```python
from build123d import *

# Parameters (mm, degrees)
EXTRUDE_1_DEPTH     = 3
SKETCH_2_W          = 112
SKETCH_2_H          = 45
CUT_EXTRUDE_1_DEPTH = 174.386325559


with BuildPart() as part:
    # Эскиз1 → Бобышка-Вытянуть1 (new body)
    with BuildSketch(Plane(origin=(0, 0, 0), x_dir=(1, 0, 0), z_dir=(0, 1, 0))):
        with BuildLine():
            Line((0, 0), (138, 0))
            Line((138, 0), (138, -68))
            ThreePointArc((138, -68), (69, -104.927679336), (0, -68))
            Line((0, -68), (0, 0))
        make_face()
    extrude(amount=EXTRUDE_1_DEPTH)

    # Эскиз2 → Вырез-Вытянуть1 (cut, through all)
    with BuildSketch(Plane(origin=(0, 3, 0), x_dir=(1, 0, 0), z_dir=(0, 1, 0))):
        with Locations((69, -31.5)):
            Rectangle(SKETCH_2_W, SKETCH_2_H)
    extrude(amount=-CUT_EXTRUDE_1_DEPTH, mode=Mode.SUBTRACT)

    # Эскиз3 → Зенковка для  винта с плоской головкой M51 (revolve, cut)
    with BuildSketch(Plane(origin=(69, 3, 82.6), x_dir=(0, 0, 1), z_dir=(1, 0, 0))):
        Polygon((0, 0), (0, 3), (2.75, 3), (2.75, 2.45), (5.2, 0), align=None)
    revolve(axis=Axis((69, 9.35, 82.6), (0, -1, 0)), mode=Mode.SUBTRACT)


solid = part.part
```
CAD build for the part. Positions are in the model's coordinates, mm. A direction names the side the tool comes from. Give positions to 0.01 mm unless a question says otherwise; leave off trailing zeros. Loops run counter-clockwise (first coordinate to the right, second up) from the corner with the lowest first, then second, coordinate; pieces in that order, holes last. Notation, with made-up numbers: M 18,22 L 73,22 A20 ccw 73,33 Z; hole C -8,-35 d6. An arc over 180 degrees is marked long. Use one line per item in the form item = value.
Item 1: Drill centre lines: probe 1 along X at (y, z) = (1, 39.5); probe 2 along Z at (x, y) = (80, 0.6); probe 3 along X at (y, z) = (0.4, 82.6). Where is each one in solid material? Low to high. Write a range as from..to.
Determined:
probe_1 = 0..13, 125..138
probe_2 = 0..9, 54..104.19
probe_3 = 12.39..66.25, 71.75..125.61
Item 2: Which spindle directions (+Z, -Z, +X, -X, +Y, -Y) get a long thin tool onto all of the face, cutting with end or side? Do faces 1 (the face through (125, 2, 32)), 2 (the face through (70, 3, 63)). Say none if no direction does.
Determined:
face_1 = +Y, -Y
face_2 = +Z, -Z, +X, -X, +Y
Item 3: Slice it at D-D (x = 103). List the corners of the cut face in (y, z), plus the area to 3 significant figures.
Determined:
outline = M 0,0 L 3,0 L 3,9 L 0,9 Z; M 0,54 L 3,54 L 3,97.64 L 0,97.64 Z
area = 158 mm2
Item 4: Slice it at A-A (z = 20). List the corners of the cut face in (x, y).
Determined:
outline = M 0,0 L 13,0 L 13,3 L 0,3 Z; M 125,0 L 138,0 L 138,3 L 125,3 Z
Item 5: Slice it at C-C (y = 2.45). List the corners of the cut face in (x, z), plus the area to 3 significant figures.
Determined:
outline = M 0,0 L 138,0 L 138,68 A82.93 ccw 0,68 Z; hole M 13,9 L 125,9 L 125,54 L 13,54 Z; hole C 69,82.6 d9.3
area = 7,860 mm2
Item 6: Two-plate mould, pull along X, no slides. Class faces 3 (the face through (70, 0, 63)), 4 (the face through (70.14, 1.48, 104.92)), 5 (the face through (68, 2, 9)): pulls with the +X half, pulls with the -X half, needs draft (parallel to the pull), parting line crosses it, or undercut.
Determined:
face_3 = needs draft
face_4 = parting line crosses it
face_5 = undercut
Item 7: Slice it at B-B (x = 69). List the corners of the cut face in (y, z), plus the area to 3 significant figures.
Determined:
outline = M 0,0 L 3,0 L 3,9 L 0,9 Z; M 0,54 L 3,54 L 3,77.4 L 0.55,79.85 L 0,79.85 Z; M 0,85.35 L 0.55,85.35 L 3,87.8 L 3,104.93 L 0,104.93 Z
area = 157 mm2
